Autodesk Inventor part; units mm, degrees
ref_plane "YZ Plane" through (0, 0, 0) normal (1, 0, 0) x (0, 1, 0)
ref_plane "XZ Plane" through (0, 0, 0) normal (0, 1, 0) x (-1, 0, 0)
ref_plane "XY Plane" through (0, 0, 0) normal (0, 0, 1) x (1, 0, 0)
ref_plane "Work Plane1" through (64.8465, 16.6938, -6.1656) normal (0, 1, 0) x (1, 0, 0)
sketch "Sketch1" plane through (64.8465, 16.6938, -6.1656) normal (0, 1, 0) x (1, 0, 0)
  line L0 (1.7321, 1) -> (27.6872, 15.9852) construction
  line L1 (13.1559, 10.8634) -> (20.3785, 15.0334)
  line L2 (15.9859, 5.9616) -> (23.2085, 10.1316)
  line L3 (13.1559, 10.8634) -> (15.9859, 5.9616)
  circle A0 centre (1.7321, 1) radius 20 construction
  circle A1 centre (19.0526, 11) radius 5.175 construction
  circle A2 centre (1.7321, 1) radius 1.5
  line L4 (1.7321, 1) -> (8.6603, 5) construction
  circle A3 centre (8.6603, 5) radius 1.5
  line L5 (17.3785, 20.2295) -> (1.7321, 11.196)
  line L6 (1.7321, 11.196) -> (-13.9144, 20.2295)
  line L7 (26.2085, 4.9355) -> (10.5621, -4.098)
  circle A4 centre (1.7321, 1) radius 10.196 construction
  line L8 (-12.5218, 5.9616) -> (-19.7444, 10.1316)
  line L9 (-9.6918, 10.8634) -> (-16.9144, 15.0334)
  line L10 (-12.5218, 5.9616) -> (-9.6918, 10.8634)
  circle A5 centre (-5.1962, 5) radius 1.5
  line L11 (4.5621, -13.825) -> (4.5621, -22.165)
  line L12 (-1.0979, -13.825) -> (-1.0979, -22.165)
  line L13 (4.5621, -13.825) -> (-1.0979, -13.825)
  circle A6 centre (1.7321, -7) radius 1.5
  line L14 (-7.0979, -22.165) -> (-7.0979, -4.098)
  line L15 (10.5621, -22.165) -> (10.5621, -4.098)
  line L16 (-7.0979, -4.098) -> (-22.7444, 4.9355)
  line L17 (-7.0979, -22.165) -> (-1.0979, -22.165)
  line L18 (4.5621, -22.165) -> (10.5621, -22.165)
  line L19 (-13.9144, 20.2295) -> (-16.9144, 15.0334)
  line L20 (-19.7444, 10.1316) -> (-22.7444, 4.9355)
  line L21 (17.3785, 20.2295) -> (20.3785, 15.0334)
  line L22 (23.2085, 10.1316) -> (26.2085, 4.9355)
  dimension "d34" = 40
  dimension "d35" = 10.35
  dimension "d45" = 3
  dimension "d47" = 8
  dimension "d48" = 3
  dimension "d54" = 360
extrude "Extrusion2" add sketch "Sketch1" along normal blind 5.66
fillet "Fillet1" radius 3 3 edges at (75.4086, 19.5238, -2.0676) (66.5786, 19.5238, -17.3616) (57.7486, 19.5238, -2.0676)
fillet "Fillet2" radius 3 2 edges at (91.055, 19.5238, -11.1011) (82.225, 19.5238, -26.3951)
pattern_circular "Circular Pattern1" count 3 over 360 about axis through (66.5786, 16.6938, -7.1656) along (0, 1, 0) of "Fillet2"
properties part number "Lower PlatformV"
Source: CAD feature listing. Evaluate the final solid. Frame: model axes, mm. A direction names the side the tool comes from. Coordinates: 2 decimals unless noted, no trailing zeros. Order: outer loops, then holes, each group sorted by start corner. A loop starts at its lowest first (then second) coordinate and runs counter-clockwise, first axis right, second up. Notation, with made-up numbers: M 21,39.25 L 67,39.25 A23 ccw 67,69.25 Z; hole C 45.5,-5 d11. An arc over 180 degrees is marked long. Write each question's results on one line, items separated by ' | '. Start each with the question number.
1. Section B-B, the plane y = 21.7. State how many separate pieces and enclosed holes the cut face has, then the cut area to 3 significant figures.
2. Draft query along X for faces 1 (the face through (67, 19, 7.659)), 2 (the face through (88.794, 19.484, -15.016)), 3 (the face through (51.594, 19.484, -19.085)). Return one class per face: +X half, -X half, draft (parallel to the pull), parting line (faces both ways), or undercut.
3. Section A-A, the plane z = 12. Return the cut outline in (x, y), then the cut area to 3 significant figures.
4. Pin query (flat end, axial travel): pin 1 (1.7 mm diameter, centred on y = 19.5, z = 9, fed in from -X); pin 2 (1.8 mm diameter, centred on x = 66.58, z = 0.83, fed in from +Y); pin 3 (1.5 mm diameter, centred on y = 19, z = -10, fed in from +X); pin 4 (2 mm diameter, centred on y = 18.5, z = -10.5, fed in from -X). Return the tip coordinate at first contact, or that it passes through.
5. Section C-C, the plane x = 84.5. Return the cut outline in (y, z).
6. Reachability of faces 4 (the face through (73.934, 19.484, -21.608)), 5 (the face through (75.409, 19, 6)), 6 (the face through (57.749, 19, 6)), 7 (the face through (84.39, 19.48, -14.18)), 8 (the face through (69.409, 19, 12)) from +Z, -Z, +X, -X, +Y, -Y: full face, straight path, thin tool, end or side. Return the list, or none.
7. Section D-D, the plane z = -15.5. Return the cut outline in (x, y), then the cut area to 3 significant figures.
8. Material intervals for L1, parallel to Z at x = 66.5, y = 21.5; L2, parallel to X at y = 17.25, z = 9.5; L3, parallel to Z at x = 67, y = 20.3, sorted ascending.
Solution:
1) separate pieces: 1 | enclosed holes: 4 | area: 912 mm²
2) face 1: undercut | face 2: +X half | face 3: -X half
3) outline: M 57.75,16.69 L 63.75,16.69 L 63.75,22.35 L 57.75,22.35 Z; M 69.41,16.69 L 75.41,16.69 L 75.41,22.35 L 69.41,22.35 Z | area: 67.9 mm²
4) pin 1: x = 57.75 | pin 2: through | pin 3: x = 89.58 | pin 4: x = 43.28
5) outline: M 16.69,-22.45 L 22.35,-22.45 L 22.35,-20.78 L 16.69,-20.78 Z; M 16.69,-14.24 L 22.35,-14.24 L 22.35,-7.32 L 16.69,-7.32 Z
6) face 4: -Z, +Y, -Y | face 5: +Z, +X, +Y, -Y | face 6: +Z, -X, +Y, -Y | face 7: +Y, -Y | face 8: +Z, +Y, -Y
7) outline: M 44.64,16.69 L 46.48,16.69 L 46.48,22.35 L 44.64,22.35 Z; M 54.27,16.69 L 78.89,16.69 L 78.89,22.35 L 54.27,22.35 Z; M 86.67,16.69 L 88.52,16.69 L 88.52,22.35 L 86.67,22.35 Z | area: 160 mm²
8) L1: -17.83 to -8.66, -5.67 to -0.66, 2.33 to 7.66 | L2: 57.75 to 63.75, 69.41 to 75.41 | L3: -17.86 to -8.61, -5.73 to -0.61, 2.27 to 7.66
